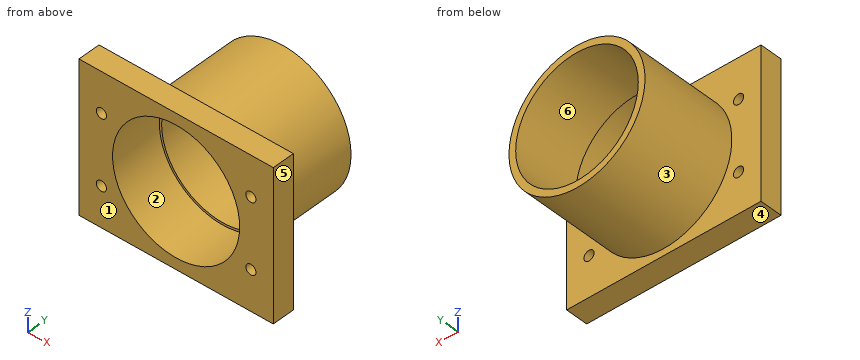
```python
from build123d import *

# Parameters (mm, degrees)
SKETCH1_W             = 130
SKETCH1_H             = 100
BOSS_EXTRUDE1_DEPTH   = 15
SKETCH2_R             = 45.5
BOSS_EXTRUDE2_DEPTH   = 65
SKETCH3_R             = 41
CUT_EXTRUDE1_DEPTH    = 81
SKETCH4_R             = 42.5
CUT_EXTRUDE2_DEPTH    = 35
M8_TAPPED_HOLE1_D     = 6.8
M8_TAPPED_HOLE1_DEPTH = 17.707073895
M8_TAPPED_HOLE1_TIP   = 2.042926105


with BuildPart() as part:
    # Sketch1 → Boss-Extrude1 (new body)
    with BuildSketch(Plane(origin=(0, 0, 0), x_dir=(1, 0, 0), z_dir=(0, 1, 0))):
        Rectangle(SKETCH1_W, SKETCH1_H)
    extrude(amount=BOSS_EXTRUDE1_DEPTH)

    # Sketch2 → Boss-Extrude2 (add)
    with BuildSketch(Plane(origin=(0, 15, 0), x_dir=(1, 0, 0), z_dir=(0, 1, 0))):
        Circle(SKETCH2_R)
    extrude(amount=BOSS_EXTRUDE2_DEPTH)

    # Sketch3 → Cut-Extrude1 (cut, through all)
    with BuildSketch(Plane(origin=(0, 80, 0), x_dir=(1, 0, 0), z_dir=(0, 1, 0))):
        Circle(SKETCH3_R)
    extrude(amount=-CUT_EXTRUDE1_DEPTH, mode=Mode.SUBTRACT)

    # Sketch4 → Cut-Extrude2 (cut)
    with BuildSketch(Plane.XZ):
        Circle(SKETCH4_R)
    extrude(amount=-CUT_EXTRUDE2_DEPTH, mode=Mode.SUBTRACT)

    # M8 Tapped Hole1
    with Locations(Plane(origin=(0, 15, 0), x_dir=(1, 0, 0), z_dir=(0, 1, 0))):
        with Locations((-50, 23.25), (-50, -23.25), (50, -23.25), (50, 23.25)):
            Hole(M8_TAPPED_HOLE1_D / 2, depth=M8_TAPPED_HOLE1_DEPTH)
            with Locations((0, 0, -(M8_TAPPED_HOLE1_DEPTH + M8_TAPPED_HOLE1_TIP / 2))):  # 118° drill point
                Cone(0, M8_TAPPED_HOLE1_D / 2, M8_TAPPED_HOLE1_TIP, mode=Mode.SUBTRACT)


solid = part.part
```
Verification items for the finished model (mm, model axes). Face numbers are marked on the shaded views. A direction names the side the tool comes from. Coordinates: 2 decimals unless noted, no trailing zeros. Write each loop counter-clockwise with the first axis right and the second up, starting at its lowest first coordinate (ties: lowest second). Pieces come first, ordered by that corner, then holes. Notation, with made-up numbers: M -31,-19 L -6,-19 A17 ccw -6,14 Z; hole C -4,70 d4. An arc over 180 degrees is marked long. Answer as a JSON object with one key per item and string values. Group by question number.
(1) Cross-section at C-C, the plane x = 4. Record the cut outline in (y, z).
(2) Cross-section at A-A, the plane x = 50. Record the cut outline in (y, z).
(3) Cross-section at B-B, the plane z = 0. Record the cut outline in (x, y).
(4) Material ranges on line 1 (Z direction, x = -50, y = 10.5); line 2 (X direction, y = 7, z = -23); line 3 (Z direction, x = 0, y = 13), recorded low to high.
(5) Release check for a two-part mould opening along Z. For the marked faces 4, 5 and 6 record: +Z half, -Z half, draft (parallel to the pull), parting line (faces both ways), or undercut.
(6) Cross-section at D-D, the plane z = -23.25. Record the cut outline in (x, y), and give its area (3 significant figures).
(7) Tool access check on the marked faces 1, 2 and 3. Record the directions out of +Z, -Z, +X, -X, +Y, -Y that give a thin tool (end or side, any length) a straight path to the whole face; none if there is none.
(8) Gauge pin test, flat ends, axial feed: pin 1 (6 mm diameter, centred on y = 28.5, z = -36.5, fed in from +X); pin 2 (12 mm diameter, centred on y = 37, z = 17, fed in from -X); pin 3 (4 mm diameter, centred on x = 35, z = -17, fed in from -Y); pin 4 (9 mm diameter, centred on x = -50, z = -23.25, fed in from +Y). Record the tip position at first contact, or that the pin passes through.
Reply:
{
 "1": {"outline": "M 0,-50 L 15,-50 L 15,-45.32 L 80,-45.32 L 80,-40.8 L 35,-40.8 L 35,-42.31 L 0,-42.31 Z; M 0,42.31 L 35,42.31 L 35,40.8 L 80,40.8 L 80,45.32 L 15,45.32 L 15,50 L 0,50 Z"},
 "2": {"outline": "M 0,-50 L 15,-50 L 15,-26.65 L 0,-26.65 Z; M 0,-19.85 L 15,-19.85 L 15,19.85 L 0,19.85 Z; M 0,26.65 L 15,26.65 L 15,50 L 0,50 Z"},
 "3": {"outline": "M -65,0 L -42.5,0 L -42.5,35 L -41,35 L -41,80 L -45.5,80 L -45.5,15 L -65,15 Z; M 41,35 L 42.5,35 L 42.5,0 L 65,0 L 65,15 L 45.5,15 L 45.5,80 L 41,80 Z"},
 "4": {"line 1": "-50 to -26.65, -19.85 to 19.85, 26.65 to 50", "line 2": "-65 to -53.39, -46.61 to -35.74, 35.74 to 46.61, 53.39 to 65", "line 3": "-50 to -42.5, 42.5 to 50"},
 "5": {"face 4": "-Z half", "face 5": "draft", "face 6": "undercut"},
 "6": {"outline": "M -65,0 L -53.4,0 L -53.4,15 L -65,15 Z; M -46.6,0 L -35.58,0 L -35.58,35 L -33.77,35 L -33.77,80 L -39.11,80 L -39.11,15 L -46.6,15 Z; M 33.77,35 L 35.58,35 L 35.58,0 L 46.6,0 L 46.6,15 L 39.11,15 L 39.11,80 L 33.77,80 Z; M 53.4,0 L 65,0 L 65,15 L 53.4,15 Z", "area": "1,300 mm²"},
 "7": {"face 1": "+Z, -Z, +X, -X, -Y", "face 2": "-Y", "face 3": "+Y"},
 "8": {"pin 1": "x = 30.79", "pin 2": "x = -44.15", "pin 3": "through", "pin 4": "y = 15"}
}
